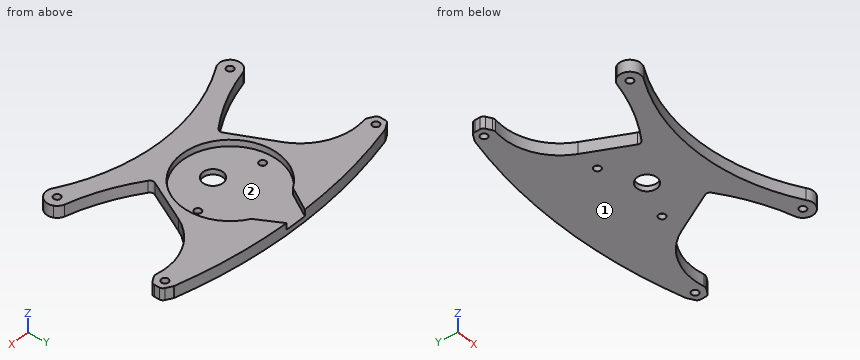
Autodesk Inventor part; units mm, degrees
ref_plane "YZ Plane" through (0, 0, 0) normal (1, 0, 0) x (0, 1, 0)
ref_plane "XZ Plane" through (0, 0, 0) normal (0, 1, 0) x (-1, 0, 0)
ref_plane "XY Plane" through (0, 0, 0) normal (0, 0, 1) x (1, 0, 0)
sketch "スケッチ1" plane through (0, 0, 0) normal (0, 0, 1) x (1, 0, 0)
  circle A0 centre (19.2131, 26.9091) radius 1.6
  circle A1 centre (8.9167, 85.9091) radius 1.6
  circle A2 centre (122.9167, 85.9091) radius 1.6
  circle A3 centre (112.6203, 26.909) radius 1.6
  line L0 (65.9168, 92.271) -> (65.9166, 46.271)
  line L1 (7.2067, 85.9091) -> (10.6267, 85.9091)
  line L2 (8.9167, 84.1991) -> (8.9167, 87.6191)
  line L3 (124.6267, 85.9091) -> (121.2067, 85.9091)
  line L4 (122.9167, 84.1991) -> (122.9167, 87.6191)
  line L5 (6.0567, 82.7816) -> (8.3869, 81.4363)
  line L6 (5.0567, 86.8043) -> (5.0567, 84.5137)
  line L7 (123.7023, 81.4412) -> (126.0241, 82.7816)
  circle A4 centre (65.9167, 59.1833) radius 4.65
  circle A5 centre (65.9167, 67.1833) radius 14
  line L8 (82.734, 67.2168) -> (82.7592, 67.2168)
  circle A6 centre (48.4167, 67.2168) radius 1.6
  circle A7 centre (83.4167, 67.2168) radius 1.6
  arc A8 (37.9167, 67.2167) -> (9.7534, 81.2022) centre (14.5444, 55.5004) ccw
  arc A9 (122.3194, 81.2102) -> (93.9167, 67.2168) centre (117.3134, 55.5494) ccw
  line L9 (37.9167, 67.2167) -> (47.5918, 47.9164)
  line L10 (93.9167, 67.2168) -> (84.2485, 47.9303)
  arc A10 (46.8453, 45.3126) -> (47.5918, 47.9164) centre (45.8039, 47.0201) ccw
  arc A11 (84.2485, 47.9303) -> (85.0094, 45.3179) centre (86.0364, 47.034) ccw
  circle A12 centre (19.2131, 26.9091) radius 1.6
  circle A13 centre (112.6203, 26.909) radius 1.6
  circle A14 centre (122.9167, 85.9091) radius 1.6
  circle A15 centre (8.9167, 85.9091) radius 1.6
  arc A16 (122.7823, 90.3275) -> (9.2985, 90.3275) centre (66.0404, -124.0864) ccw
  arc A17 (123.2706, 90.1261) -> (122.7823, 90.3275) centre (122.2706, 88.394) ccw
  arc A18 (126.0241, 82.7816) -> (127.0241, 84.5137) centre (125.0241, 84.5137) ccw
  arc A19 (122.3194, 81.2102) -> (123.7023, 81.4412) centre (122.7023, 83.1732) ccw
  arc A20 (9.2985, 90.3275) -> (8.8102, 90.1261) centre (9.8102, 88.394) ccw
  arc A21 (8.3869, 81.4363) -> (9.7534, 81.2022) centre (9.3869, 83.1683) ccw
  arc A22 (6.0567, 88.5363) -> (5.0567, 86.8043) centre (7.0567, 86.8043) ccw
  arc A23 (5.0567, 84.5137) -> (6.0567, 82.7816) centre (7.0567, 84.5137) ccw
  line L11 (8.8102, 90.1261) -> (6.0567, 88.5363)
  line L12 (123.2706, 90.1261) -> (126.0241, 88.5363)
  line L13 (127.0241, 84.5137) -> (127.0241, 86.8043)
  arc A24 (127.0241, 86.8043) -> (126.0241, 88.5363) centre (125.0241, 86.8043) ccw
  arc A25 (14.749, 29.1208) -> (22.1634, 22.8946) centre (19.2131, 26.9091) ccw
  arc A26 (109.6696, 22.8946) -> (117.0846, 29.1208) centre (112.6203, 26.909) ccw
  arc A27 (109.6696, 22.8946) -> (22.1634, 22.8946) centre (65.9165, -52.1885) ccw
  arc A28 (18.2456, 31.7962) -> (22.1634, 22.8946) centre (19.2131, 26.9091) ccw
  arc A29 (109.6696, 22.8946) -> (113.5922, 31.7955) centre (112.6203, 26.909) ccw
  arc A30 (17.6131, 31.6271) -> (46.8453, 45.3126) centre (-5.3123, 118.6583) ccw
  arc A31 (85.0094, 45.3179) -> (114.2208, 31.6271) centre (137.191, 118.6465) ccw
  point P0 (0, 0)
  dimension "d10" = 28
  dimension "d13" = 17.5
  dimension "d15" = 17.5
  dimension "d20" = 3.2
  dimension "d27" = 2.681
  dimension "d28" = 2.2906
  dimension "d29" = 2
  dimension "d31" = 2.2906
  dimension "d35" = 46.7037
  dimension "d36" = 46.7035
  dimension "d39" = 90
  dimension "d40" = 90
extrude "押し出し1" add sketch "スケッチ1" along normal blind 5.5 contours A5 L0 A4 | L0 A4 A5 | A23 L6 A22 L11 A20 A16 A17 L12 A24 L13 A18 L7 A19 A9 L10 A11 A31 A29 A26 A27 A25 A28 A30 A10 L9 A8 A21 L5
sketch "スケッチ3" plane through (0, 0, 5.5) normal (0, 0, 1) x (1, 0, 0)
  circle A0 centre (48.4167, 67.2168) radius 1.6
  circle A1 centre (83.4167, 67.2168) radius 1.6
  arc A2 (54.6667, 86.7024) -> (77.1667, 86.7024) centre (65.9167, 67.2168) ccw
  line L0 (54.6667, 86.7024) -> (60.9878, 97.6509)
  arc A3 (122.7823, 90.3275) -> (9.2985, 90.3275) centre (66.0404, -124.0864) ccw
  line L1 (77.1667, 86.7024) -> (70.8424, 97.6564)
  arc A4 (70.8424, 97.6564) -> (60.9878, 97.6509) centre (66.0404, -124.0864) ccw
  line L2 (60.9878, 97.6509) -> (54.6667, 86.7024)
  arc A5 (70.8424, 97.6564) -> (60.9878, 97.6509) centre (66.0404, -124.0864) ccw
  line L3 (70.8424, 97.6564) -> (77.1667, 86.7024)
  point P0 (0, 0)
extrude "押し出し2" cut sketch "スケッチ3" against normal blind 3
properties part number "ステッピング固定具" material "MDF 中密度繊維ボード"
Can you work these out from the model? Positions are in its coordinate system, mm. Face numbers are marked on the shaded views. Round coordinates to 2 decimals unless told otherwise and drop trailing zeros. Write each loop counter-clockwise with the first axis right and the second up, starting at its lowest first coordinate (ties: lowest second). Pieces come first, ordered by that corner, then holes. Notation, with made-up numbers: (50, -27.5) - (59, -27.5) arc R19 ccw to (59, -11.5) - close; hole circle Ø10 at (-39.75, 75.25). An arc over 180 degrees is marked (long way). Write each question's results on one line, items separated by ' | '. Start each with the question number.
1) We'd pull the mould along X, two halves only. Please class the marked faces 1 and 2: released by +X, released by -X, zero draft, split by the parting line, or undercut.
2) Suppose I cut it at A-A (x = 29). List the corners of the cut face in (y, z) for me, and give its area (3 significant figures).
3) Suppose I cut it at D-D (z = 3.6). Give the number of separate pieces and of enclosed holes in the cut face, and give its area (3 significant figures).
4) Suppose I cut it at C-C (x = 99.5). List the corners of the cut face in (y, z) for me, and give its area (3 significant figures).
5) For pin 1 Ø3 at (x, y) = (19.21, 26.91) entering from +Z; pin 2 Ø1 at (x, z) = (77.5, 0.5) entering from -Y; pin 3 Ø1 at (x, z) = (62.5, 4) entering from -Y; pin 4 Ø2 at (y, z) = (63.5, 3) entering from +X, each with a flat end and sliding along its axis, tell me the tip position at first contact or that it passes through.
6) Please list where these lines run through material, in increasing order: line 1 (Z direction, x = 48.5, y = 65); line 2 (X direction, y = 86.5, z = 0.8); line 3 (Y direction, x = 32.5, z = 2.25).
7) Suppose I cut it at B-B (y = 56). List the corners of the cut face in (x, z) for me, and give its area (3 significant figures).
Here are the results:
1) face 1: zero draft | face 2: undercut
2) outline: (26.48, 0) - (35.46, 0) - (35.46, 5.5) - (26.48, 5.5) - close; (77.29, 0) - (94.59, 0) - (94.59, 5.5) - (77.29, 5.5) - close | area: 145 mm2
3) separate pieces: 1 | enclosed holes: 4 | area: 2,900 mm2
4) outline: (27.96, 0) - (36.92, 0) - (36.92, 5.5) - (27.96, 5.5) - close; (74.69, 0) - (95.17, 0) - (95.17, 5.5) - (74.69, 5.5) - close | area: 162 mm2
5) pin 1: passes through | pin 2: stops at y = 33.87 | pin 3: stops at y = 34.62 | pin 4: stops at x = 92.55
6) line 1: z = 0 to 2.5 | line 2: x = 5.06 to 7.43, 10.4 to 121.43, 124.4 to 127.02 | line 3: y = 28.03 to 36.99, 74.5 to 95.16
7) outline: (43.54, 0) - (62.53, 0) - (62.53, 2.5) - (46.41, 2.5) - (46.41, 5.5) - (43.54, 5.5) - close; (69.31, 0) - (88.29, 0) - (88.29, 5.5) - (85.42, 5.5) - (85.42, 2.5) - (69.31, 2.5) - close | area: 112 mm2
